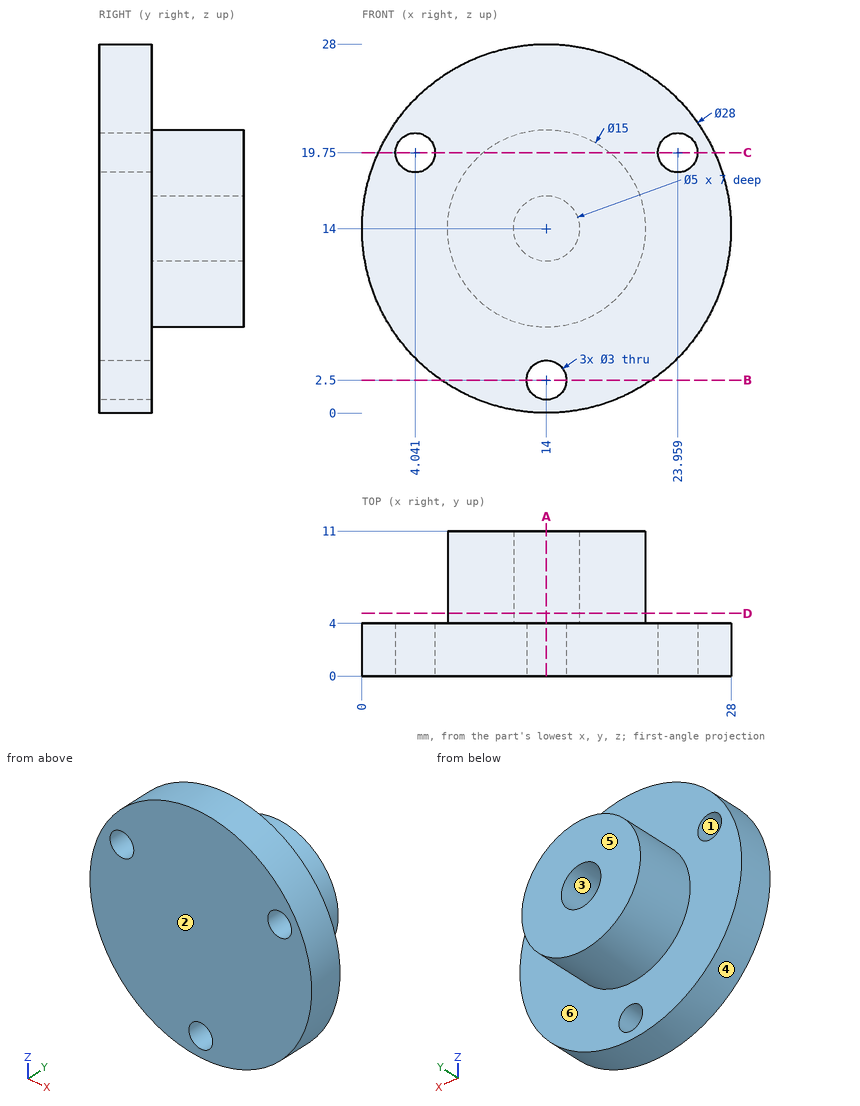
Input: dimensioned drawing with shaded views. Units: mm. Origin: part minimum x, y, z. A direction names the side the tool comes from. Give positions to 0.01 mm unless a question says otherwise; leave off trailing zeros. Loops run counter-clockwise (first coordinate to the right, second up) from the corner with the lowest first, then second, coordinate; pieces in that order, holes last. Notation, with made-up numbers: (18, 42) -> (75, 42) arc R19 cw to (75, 69) -> close; hole circle Ø11 at (27, 83). An arc over 180 degrees is marked (long way). Use a Markdown table: item, result. Add a question column.
1) Pull-direction query (Z, two-part tool) for the marked faces 1, 2, 3 and 4; classes: +Z half, -Z half, draft (parallel to the pull), parting line (faces both ways), or undercut.
2) Line query: line 1 along X through (y, z) = (1, 20.25) (1 decimal); line 2 along X through (y, z) = (7, 14); line 3 along Y through (x, z) = (22.75, 18.25). Output: solid intervals per line, ascending. Write a range as [from, to].
3) Section query D-D, the plane y = 4.75. Return the cut outline in (x, z).
4) Section query A-A, the plane x = 14. Return the cut outline in (y, z).
5) Reachability of the marked faces 5 and 6 from +Z, -Z, +X, -X, +Y, -Y: full face, straight path, thin tool, end or side. Return the list, or none.
6) First-contact query: pin 1 (3.5 mm diameter, centred on x = 23.96, z = 19.75, fed in from +Y); pin 2 (1 mm diameter, centred on x = 4, y = 3.5, fed in from +Z); pin 3 (5 mm diameter, centred on x = 10, y = 8, fed in from +Z); pin 4 (2.5 mm diameter, centred on x = 14, z = 2.5, fed in from +Y). Flat tips, straight axial feed; report the tip coordinate or a pass-through.
7) Section query B-B, the plane z = 2.5. Return the cut outline in (x, y).
8) Section query C-C, the plane z = 19.75. Return the cut outline in (x, y) (1 decimal).
Numbers:
| question | item | result |
|---|---|---|
| 1 | face 1 | undercut |
| 1 | face 2 | draft |
| 1 | face 3 | undercut |
| 1 | face 4 | parting line |
| 2 | line 1 | x = [1.5, 2.6], [5.5, 22.5], [25.4, 26.5] |
| 2 | line 2 | x = [6.5, 11.5], [16.5, 21.5] |
| 2 | line 3 | y = [0, 4] |
| 3 | outline | circle Ø15 at (14, 14); hole circle Ø5 at (14, 14) |
| 4 | outline | (0, 0) -> (4, 0) -> (4, 1) -> (0, 1) -> close; (0, 4) -> (4, 4) -> (4, 6.5) -> (11, 6.5) -> (11, 11.5) -> (4, 11.5) -> (4, 16.5) -> (11, 16.5) -> (11, 21.5) -> (4, 21.5) -> (4, 28) -> (0, 28) -> close |
| 5 | face 5 | +Z, -Z, +X, -X, +Y |
| 5 | face 6 | +Y |
| 6 | pin 1 | stops at y = 4 |
| 6 | pin 2 | stops at z = 24.28 |
| 6 | pin 3 | stops at z = 21.35 |
| 6 | pin 4 | passes through |
| 7 | outline | (6.02, 0) -> (12.5, 0) -> (12.5, 4) -> (6.02, 4) -> close; (15.5, 0) -> (21.98, 0) -> (21.98, 4) -> (15.5, 4) -> close |
| 8 | outline | (1.2, 0) -> (2.5, 0) -> (2.5, 4) -> (1.2, 4) -> close; (5.5, 0) -> (22.5, 0) -> (22.5, 4) -> (18.8, 4) -> (18.8, 11) -> (9.2, 11) -> (9.2, 4) -> (5.5, 4) -> close; (25.5, 0) -> (26.8, 0) -> (26.8, 4) -> (25.5, 4) -> close |
